```python
from build123d import *

# Parameters (mm, degrees)
SKETCH024_R          = 1.25
POCKET007_DEPTH      = 12.001
PAD001_DEPTH         = 2.5
POCKET008_DEPTH      = 7.5
POCKET008_DEPTH_BACK = 100


with BuildPart() as part:
    # Sketch023 → Revolution001 (revolve)
    with BuildSketch(Plane.YZ):
        with BuildLine():
            Line((0, 0), (0, 12))
            Line((0, 12), (13, 12))
            ThreePointArc((5, 0), (10.816654, 4.788897), (13, 12))
            Line((0, 0), (5, 0))
        make_face()
    revolve(axis=Axis((0, 0, 0), (0, 0, 1)))

    # Sketch024 → Pocket007 (cut, through all)
    with BuildSketch(Plane.XY):
        Circle(SKETCH024_R)
    extrude(amount=POCKET007_DEPTH, mode=Mode.SUBTRACT)

    # Sketch025 (on DatumPlane) → Pad001 (join, symmetric)
    with BuildSketch(Plane(origin=(0, 0, 12), x_dir=(0, 1, 0), z_dir=(1, 0, 0))):
        with BuildLine():
            ThreePointArc((-3.3, 4.5), (-3.55, 4.25), (-3.3, 4))
            Line((-3.3, 4), (-3.3, 1))
            Line((-3.3, 1), (-4.3, 0))
            Line((-4.3, 0), (-1.5, 0))
            Line((-1.5, 0), (-2.5, 1))
            Line((-2.5, 4.5), (-2.5, 1))
            Line((-3.3, 4.5), (-2.5, 4.5))
        make_face()
        with BuildLine():
            Line((4.3, 0), (1.5, 0))
            Line((2.5, 1), (1.5, 0))
            Line((2.5, 4.5), (2.5, 1))
            Line((3.3, 4.5), (2.5, 4.5))
            ThreePointArc((3.3, 4), (3.55, 4.25), (3.3, 4.5))
            Line((3.3, 1), (3.3, 4))
            Line((4.3, 0), (3.3, 1))
        make_face()
    extrude(amount=PAD001_DEPTH, both=True)

    # Sketch026 (on DatumPlane) → Pocket008 (cut, two sides)
    with BuildSketch(Plane.XY.offset(10)) as pocket008_sk:
        Polygon((1.212436, -2.1), (2.424871, 0), (1.212436, 2.1), (-1.212436, 2.1), (-2.424871, 0), (-1.212436, -2.1), align=None)
    extrude(amount=-POCKET008_DEPTH, mode=Mode.SUBTRACT)
    extrude(pocket008_sk.sketch, amount=POCKET008_DEPTH_BACK, mode=Mode.SUBTRACT)


with BuildPart() as part_1:
    # Body007 placement: moved
    add(part.part.moved(Location((0, -24, 0))))


solid = part_1.part
```
Source: CAD feature listing. Evaluate the final solid. Frame: model axes, mm. A direction names the side the tool comes from. Give positions to 0.01 mm unless a question says otherwise; leave off trailing zeros. Use CSV: the item, a comma, the result in double quotes.
1) Line query: line 1 (X direction, y = -24, z = 0.95); line 2 (Y direction, x = 0, z = 0.7); line 3 (X direction, y = -23.25, z = 7.5). Output: solid intervals per line, ascending.
Worked out:
line 1,"x = -6.85 to -1.25, 1.25 to 6.85"
line 2,"y = -30.43 to -25.25, -22.75 to -17.57"
line 3,"x = -12.17 to -1.99, 1.99 to 12.17"
2) Pin query (flat end, axial travel): P1, Ø3, axis at y = -27.5, z = 14.5, coming from the +X side; P2, Ø1.5, axis at y = -22.5, z = 4.5, coming from the -X side; P3, Ø4, axis at x = 3, y = -14, coming from the +Z side; P4, Ø2, axis at x = 0, y = -24, coming from the +Z side. Return the tip coordinate at first contact, or that it passes through.
Worked out:
P1,"stops at x = 2.5"
P2,"stops at x = -11.02"
P3,"stops at z = 12"
P4,"passes through"
3) Set-up query: faces 1 (the flat face through (-1.81, -22.935, 7.479)), 2 (the flat face through (2.5, -27, 14)), 3 (the flat face through (0.04, -21.77, 12.73)), 4 (the flat face through (0, -27.3, 15)), 5 (the flat face through (-2.5, -27, 14)). Return all of +Z, -Z, +X, -X, +Y, -Y with unobstructed straight access to the full face (end or side cutting, diameter ignored); none if empty.
Worked out:
face 1,"+Z"
face 2,"+Z, +X, +Y, -Y"
face 3,"+Z, +X, -X"
face 4,"+X, -X, -Y"
face 5,"+Z, -X, +Y, -Y"
4) Mould query, pull axis Y, two halves, no side actions, for faces 6 (the flat face through (-0.04, -26.22, 12.72)), 7 (the flat face through (-1.827, -25.035, 7.479)), 8 (the flat face through (0, -20.2, 12.5)), 9 (the flat face through (-2.5, -21, 14)). Classes: +Y half, -Y half, draft (parallel to the pull), parting line (faces both ways), or undercut.
Worked out:
face 6,"undercut"
face 7,"undercut"
face 8,"+Y half"
face 9,"draft"
